For this review, take the finished solid that the model builds, in its own axes (mm). A direction names the side the tool comes from. Round coordinates to 2 decimals unless told otherwise and drop trailing zeros. Order: outer loops, then holes, each group sorted by start corner. A loop starts at its lowest first (then second) coordinate and runs counter-clockwise, first axis right, second up. Notation, with made-up numbers: (-22, 14) - (19, 14) arc R30 cw to (19, 36) - close; hole circle Ø7 at (3.25, -24.5). An arc over 180 degrees is marked (long way). One line per item, written item: value.
```python
from build123d import *

# Parameters (mm, degrees)
F2_DEPTH = 305
F3_DEPTH = 75


with BuildPart() as f1:
    # F0 (on Front) → F1 (revolve)
    with BuildSketch(Plane.XZ):
        with BuildLine():
            Line((400, 0), (0, 0))
            Line((0, 0), (0, -27))
            Line((0, -27), (1079.1214704514, -27))
            Line((1079.1214704514, -27), (1079.1214704514, 0))
            Line((1079.1214704514, 0), (579.1214704514, 0))
            ThreePointArc((579.1214704514, 0), (489.5607352257, 32.3948202648), (400, 0))
        make_face()
    revolve(axis=Axis((539.5607352257, 0, -27), (1, 0, 0)))

    # F2 (add): a face of the model
    f2_faces = [f1.faces().sort_by_distance(p)[0] for p in [
        (1079.1214704514, 0, -27),
    ]]
    extrude(f2_faces, amount=F2_DEPTH)

    # F3 (cut): a face of the model
    f3_faces = [f1.faces().sort_by_distance(p)[0] for p in [
        (0, 0, -27),
    ]]
    extrude(f3_faces, amount=-F3_DEPTH, mode=Mode.SUBTRACT)


solid = f1.part
```
Item 1: Take a section at A-A (x = 1297.5). Write out the cut boundary in (y, z).
Returned:
outline: circle Ø54 at (0, -27)
Item 2: For P1, Ø6, axis at x = 1010, y = 25, coming from the +Z side; P2, Ø1, axis at x = 1155.5, y = 13.5, coming from the -Z side; P3, Ø2, axis at x = 1030.5, y = 3, coming from the +Z side, all flat-tipped, find the tip position at first contact; note any pin that passes through.
Returned:
P1: z = -11.35
P2: z = -50.66
P3: z = -0.07
Item 3: Wall thickness on line 1 (Y direction, x = 1197.5, z = -29); line 2 (X direction, y = -43.5, z = -23); line 3 (Y direction, x = 549.5, z = -68.5): over which ranges is each line inside the solid? List them lowest first.
Returned:
line 1: -26.93 to 26.93
line 2: 425.12 to 554
line 3: -19.64 to 19.64
Item 4: Machinability: for faces 1 (the cylindrical face through (235.22, 10.34, -2.06)), 2 (the flat face through (1384.121, 0, -27)), 3 (the cylindrical face through (975.99, 10.34, -2.06)), which of the approach directions +Z, -Z, +X, -X, +Y, -Y give a long, thin tool a straight path to every point of the face, cutting with its end or side? Answer none if there is none.
Returned:
face 1: -X
face 2: +Z, -Z, +X, +Y, -Y
face 3: +X
